from build123d import *

# Parameters (mm, degrees)
SKETCH1_R                            = 30.1625
EXTRUDE1_DEPTH                       = 9.3345
CIRPATTERN1_COUNT                    = 3
F_1_2_0_5_DIAMETER_HOLE1_D           = 12.69746
F_1_2_0_5_DIAMETER_HOLE1_CSINK_D     = 14.224
F_1_2_0_5_DIAMETER_HOLE1_CSINK_ANGLE = 90
CHAMFER1_SIZE                        = 0.762
F_1_2_0_5_DIAMETER_HOLE2_D           = 12.7254
F_1_2_0_5_DIAMETER_HOLE2_DEPTH       = 3.175
F_1_2_0_5_DIAMETER_HOLE2_TIP         = 3.823095861


with BuildPart() as part:
    # Sketch1 → Extrude1 (new body, symmetric)
    with BuildSketch(Plane(origin=(0, 0, 0), x_dir=(1, 0, 0), z_dir=(0, 1, 0))):
        with Locations(Location((0, 0, 0), (0, 0, 270))):  # turned: the seam where the file's is
            Circle(SKETCH1_R)
    extrude(amount=EXTRUDE1_DEPTH, both=True)

    # Sketch2 → Tapped Hole for _8-32 Helicoil1 (revolve, cut)
    with BuildSketch(Plane(origin=(0, 9.3345, -24.13), x_dir=(0, 0, 1), z_dir=(1, 0, 0))):
        Polygon((0, 0), (0, 18.669), (2.1971, 18.669), (2.1971, 10.3632), (2.63779, 10.3632), (2.63779, 0.456805306), (3.429, 0), align=None)
    tapped_hole_for_8_32_helicoil1 = revolve(axis=Axis((0, 15.6845, -24.13), (0, -1, 0)), mode=Mode.SUBTRACT)

    # CirPattern1: Tapped Hole for _8-32 Helicoil1 ×3 about axis
    cirpattern1_axis = Axis((0, 0, 0), (0, 1, 0))
    for i in range(1, CIRPATTERN1_COUNT):
        add(tapped_hole_for_8_32_helicoil1.rotate(cirpattern1_axis, i * 360 / CIRPATTERN1_COUNT), mode=Mode.SUBTRACT)

    # 1_2 _0.5_ Diameter Hole1 (through all)
    with Locations(Plane(origin=(-26.174612808, -9.3345, 9.244261036), x_dir=(1, 0, 0), z_dir=(0, -1, 0))):
        with Locations((26.174612808, -9.244261036)):
            CounterSinkHole(F_1_2_0_5_DIAMETER_HOLE1_D / 2, F_1_2_0_5_DIAMETER_HOLE1_CSINK_D / 2, counter_sink_angle=F_1_2_0_5_DIAMETER_HOLE1_CSINK_ANGLE)

    # Chamfer1
    chamfer1_edges = [part.edges().sort_by_distance(p)[0] for p in [
        (0, -9.3345, -30.1625),
        (0, 9.3345, -30.1625),
    ]]
    chamfer(chamfer1_edges, length=CHAMFER1_SIZE)

    # 1_2 _0.5_ Diameter Hole2
    with Locations(Plane.XZ.offset(9.3345)):
        with Locations((0, 0)):
            Hole(F_1_2_0_5_DIAMETER_HOLE2_D / 2, depth=F_1_2_0_5_DIAMETER_HOLE2_DEPTH)
            with Locations((0, 0, -(F_1_2_0_5_DIAMETER_HOLE2_DEPTH + F_1_2_0_5_DIAMETER_HOLE2_TIP / 2))):  # 118° drill point
                Cone(0, F_1_2_0_5_DIAMETER_HOLE2_D / 2, F_1_2_0_5_DIAMETER_HOLE2_TIP, mode=Mode.SUBTRACT)


solid = part.part
Work out the finished part from the listing and answer in its coordinate system (mm). A direction names the side the tool comes from. Give positions to 0.01 mm unless a question says otherwise; leave off trailing zeros. Loops run counter-clockwise (first coordinate to the right, second up) from the corner with the lowest first, then second, coordinate; pieces in that order, holes last. Notation, with made-up numbers: (32, 26.25) - (81, 26.25) arc R33 ccw to (81, 63.25) - close; hole circle Ø7 at (-37.5, -31.75). An arc over 180 degrees is marked (long way). Answer in a Markdown table with one row per item. Add a question column.
Q1. Consider line 1 along X through (y, z) = (5, 13); line 2 along X through (y, z) = (7.75, -23); line 3 along X through (y, z) = (4.5, -24.13). Determine where each line is inside the solid, lowest interval first.
Q2. The part is cut by section D-D (y = -7). Determine the outline of the cut face in (x, z) (1 decimal), and give its area (3 significant figures).
Q3. Determine the mould class of faces 3 (the flat face through (-6, -9.334, 6)), 4 (the cylindrical face through (1.326, 0.12, -30.133)), 5 (the cylindrical face through (0.83, -7.36, 6.31)) for opening direction X: released by +X, released by -X, zero draft, split by the parting line, or undercut.
Q4. A tool of negligible diameter and unlimited length cuts with its end or side. For faces 1 (the flat face through (7, 9.334, 0)), 2 (the cylindrical face through (18.282, 3.994, 11.722)), from which of +Z, -Z, +X, -X, +Y, -Y can it reach the whole face along a straight path? Write none if from no direction.
Q5. The part is cut by section B-B (x = 0). State how many separate pieces and enclosed holes the cut face has, and give its area (3 significant figures).
Q6. The part is cut by section C-C (y = 6.5). Determine the outline of the cut face in (x, z) (1 decimal), and give its area (3 significant figures).
Q7. Each of these flat-tipped pins is pushed along its axis until it touches: P1, Ø5, axis at y = 3, z = -22.5, coming from the +X side; P2, Ø3, axis at x = -3.5, y = 2, coming from the -Z side; P3, Ø3, axis at y = 2.5, z = -21.5, coming from the -X side. Where does it stop, or does it pass through?
Solution:
| question | item | result |
|---|---|---|
| 1 | line 1 | x = -27.22 to -23.36, -18.43 to 18.43, 23.36 to 27.22 |
| 1 | line 2 | x = -19.51 to -2.38, 2.38 to 19.51 |
| 1 | line 3 | x = -18.1 to -2.64, 2.64 to 18.1 |
| 2 | outline | circle Ø60.3 at (0, 0); hole circle Ø4.4 at (-20.9, 12.1); hole circle Ø12.7 at (0, 0); hole circle Ø4.4 at (0, -24.1); hole circle Ø4.4 at (20.9, 12.1) |
| 2 | area | 2,690 mm² |
| 3 | face 3 | zero draft |
| 3 | face 4 | split by the parting line |
| 3 | face 5 | undercut |
| 4 | face 1 | +Z, -Z, +X, -X, +Y |
| 4 | face 2 | +Y |
| 5 | separate pieces | 3 |
| 5 | enclosed holes | 0 |
| 5 | area | 796 mm² |
| 6 | outline | circle Ø60.3 at (0, 0); hole circle Ø5.3 at (-20.9, 12.1); hole circle Ø12.7 at (0, 0); hole circle Ø5.3 at (0, -24.1); hole circle Ø5.3 at (20.9, 12.1) |
| 6 | area | 2,670 mm² |
| 7 | P1 | stops at x = 22.58 |
| 7 | P2 | stops at z = -30.1 |
| 7 | P3 | stops at x = -22.58 |
